Geometry check sheet. Reference: the model listing, model coordinates, mm. Face numbers are marked on the shaded views. A direction names the side the tool comes from. Round coordinates to 2 decimals unless told otherwise and drop trailing zeros. Order: outer loops, then holes, each group sorted by start corner. A loop starts at its lowest first (then second) coordinate and runs counter-clockwise, first axis right, second up.
```python
from build123d import *

# Parameters (mm, degrees)
BOSS_EXTRUDE1_DEPTH = 60
SKETCH2_R           = 1.55
CUT_EXTRUDE1_DEPTH  = 5
SKETCH3_R           = 1.95
CUT_EXTRUDE2_DEPTH  = 5
SKETCH4_W           = 31
SKETCH4_H           = 30
CUT_EXTRUDE3_DEPTH  = 15


with BuildPart() as part:
    # Sketch1 → Boss-Extrude1 (new body)
    with BuildSketch(Plane(origin=(0, 0, 0), x_dir=(1, 0, 0), z_dir=(0, 1, 0))):
        with BuildLine():
            ThreePointArc((-44.732538493, 20), (-48.92681392, 2.677102848), (-46.647615159, -15))
            Line((-46.647615159, -15), (-41.36423576, -15))
            Line((-41.36423576, -15), (-35, -15))
            Line((-35, -15), (-35, -11))
            Line((-35, -11), (-42.602816808, -11))
            ThreePointArc((-42.602816808, -11), (-43.950159036, 2.093685925), (-41.36423576, 15))
            Line((-41.36423576, 15), (-35, 15))
            Line((-35, 15), (-35, 20))
            Line((-35, 20), (-39.191835885, 20))
            Line((-39.191835885, 20), (-44.732538493, 20))
        make_face()
    extrude(amount=BOSS_EXTRUDE1_DEPTH)

    # Sketch2 → Cut-Extrude1 (cut, through all)
    with BuildSketch(Plane(origin=(0, 0, 11), x_dir=(-1, 0, 0), z_dir=(0, 0, -1))):
        with Locations((39.997615159, 50)):
            Circle(SKETCH2_R)
        with Locations((39.997615159, 10)):
            Circle(SKETCH2_R)
    extrude(amount=-CUT_EXTRUDE1_DEPTH, mode=Mode.SUBTRACT)

    # Sketch3 → Cut-Extrude2 (cut)
    with BuildSketch(Plane(origin=(0, 0, -20), x_dir=(-1, 0, 0), z_dir=(0, 0, -1))):
        with Locations((40, 3.5)):
            Circle(SKETCH3_R)
        with Locations((40, 56.5)):
            Circle(SKETCH3_R)
    extrude(amount=-CUT_EXTRUDE2_DEPTH, mode=Mode.SUBTRACT)

    # Sketch4 → Cut-Extrude3 (cut, through all)
    with BuildSketch(Plane(origin=(-35, 0, 0), x_dir=(0, 0, -1), z_dir=(1, 0, 0))):
        with Locations((4.5, 30)):
            Rectangle(SKETCH4_W, SKETCH4_H)
    extrude(amount=-CUT_EXTRUDE3_DEPTH, mode=Mode.SUBTRACT)


solid = part.part
```
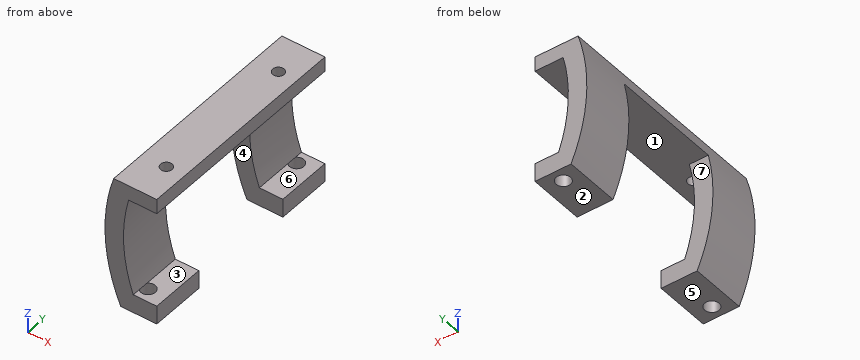
(1) Set-up check for the marked faces 1, 2, 3 and 4: record each of +Z, -Z, +X, -X, +Y, -Y from which the full face is reachable in a straight line by a thin tool's end or side.
Returned:
face 1: +X
face 2: -Z, +X, -X, +Y, -Y
face 3: +X, +Y, -Y
face 4: -Z, +X, -X
(2) Depth check by flat-ended pin: P1, Ø2, axis at y = 46, z = -10.5, coming from the +X side; P2, Ø0.6, axis at x = -41.5, y = 3.5, coming from the -Z side; P3, Ø2.5, axis at x = -40, y = 56.5, coming from the -Z side. Enter the tip coordinate at first touch or a pass-through.
Returned:
P1: stops at x = -42.47
P2: stops at z = -15
P3: stops at z = 11
(3) Sectioned sample at D-D, the plane z = -7. Record the cut outline in (x, y), and give its area (3 significant figures).
Returned:
outline: (-48.5, 0) - (-43.44, 0) - (-43.44, 15) - (-48.5, 15) - close; (-48.5, 45) - (-43.44, 45) - (-43.44, 60) - (-48.5, 60) - close
area: 152 mm2
(4) Material ranges on line 1 (Y direction, x = -40, z = -19); line 2 (Y direction, x = -48, z = -7); line 3 (Z direction, x = -40.5, y = 29), recorded low to high.
Returned:
line 1: y = 0 to 1.55, 5.45 to 15, 45 to 54.55, 58.45 to 60
line 2: y = 0 to 15, 45 to 60
line 3: z = 11 to 15
(5) Sectioned sample at A-A, the plane x = -40. Record the cut outline in (y, z).
Returned:
outline: (0, -20) - (1.55, -20) - (1.55, -15) - (0, -15) - close; (0, 11) - (8.45, 11) - (8.45, 15) - (0, 15) - close; (5.45, -20) - (15, -20) - (15, -15) - (5.45, -15) - close; (11.55, 11) - (48.45, 11) - (48.45, 15) - (11.55, 15) - close; (45, -20) - (54.55, -20) - (54.55, -15) - (45, -15) - close; (51.55, 11) - (60, 11) - (60, 15) - (51.55, 15) - close; (58.45, -20) - (60, -20) - (60, -15) - (58.45, -15) - close
(6) Draft check along Z on the marked faces 5, 6 and 7. Enter one of: released by +Z, released by -Z, zero draft, split by the parting line, or undercut.
Returned:
face 5: released by -Z
face 6: undercut
face 7: zero draft
(7) Sectioned sample at C-C, the plane y = 50. Record the cut outline in (x, z), and give its area (3 significant figures).
Returned:
outline: (-46.65, 15) arc R49 ccw to (-44.73, -20) - (-35, -20) - (-35, -15) - (-41.36, -15) arc R44 cw to (-42.6, 11) - (-41.55, 11) - (-41.55, 15) - close; (-38.45, 11) - (-35, 11) - (-35, 15) - (-38.45, 15) - close
area: 222 mm2
(8) Sectioned sample at B-B, the plane z = -12. Record the cut outline in (x, y).
Returned:
outline: (-47.51, 0) - (-42.33, 0) - (-42.33, 15) - (-47.51, 15) - close; (-47.51, 45) - (-42.33, 45) - (-42.33, 60) - (-47.51, 60) - close
